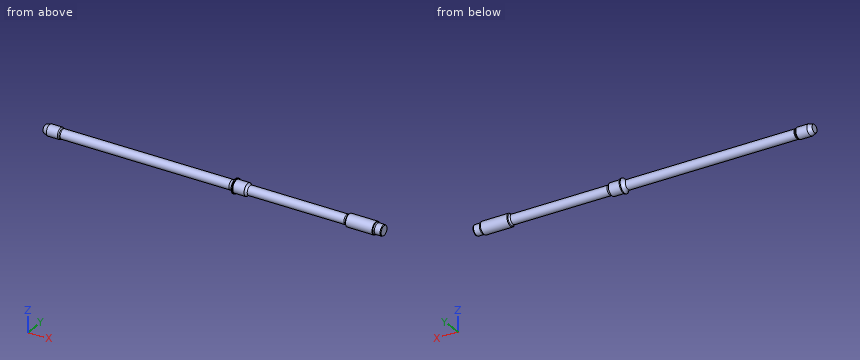
```python
from build123d import *

# Parameters (mm, degrees)
F4_R = 0.25
F5_R = 5
F6_R = 5


# Not quite as in the source:
# - a fillet or chamfer that OpenCascade refuses, or shapes differently, is made with other operations: its cross-section is extruded or revolved along the edge and cut away or added


with BuildPart() as f1:
    # F0 (on Front) → F1 (revolve)
    with BuildSketch(Plane.XZ):
        with BuildLine():
            Line((-2, 9.525), (-350.6009565311, 9.525))
            Line((-350.6009565311, 9.525), (-354, 11.11))
            Line((-354, 11.11), (-376.25, 11.11))
            Line((-376.25, 11.11), (-385, 8))
            Line((-385, 8), (-385, 0))
            Line((-385, 0), (297.49, 0))
            Line((297.49, 0), (297.49, 9.6239745962))
            Line((297.49, 9.6239745962), (295.99, 10.49))
            Line((295.99, 10.49), (284.1809884429, 10.49))
            ThreePointArc((284.1809884429, 10.49), (282.8216403227, 10.297737003), (281.7297929543, 11.13))
            Line((281.7297929543, 11.13), (280.97, 12.446))
            Line((280.97, 12.446), (227.5, 12.446))
            Line((227.5, 12.446), (224.579, 9.525))
            Line((224.579, 9.525), (23, 9.525))
            Line((23, 9.525), (23, 12.495))
            Line((23, 12.495), (0, 12.495))
            Line((0, 12.495), (0, 14.35))
            Line((0, 14.35), (-2, 14.35))
            Line((-2, 14.35), (-2, 9.525))
        make_face()
    revolve(axis=Axis((-43.755, 0, 0), (-1, 0, 0)))

    # F2: fillet of radius 8 on 1 edges, made by hand

    # F2_s1 → F2_t2 (revolve)
    with BuildSketch(Plane.XZ):
        with BuildLine():
            ThreePointArc((-2, 14.35), (-4.9498048155, 10.8391941398), (-9.3429813428, 9.525))
            Line((-9.3429813428, 9.525), (-2, 9.525))
            Line((-2, 9.525), (-2, 14.35))
        make_face()
    revolve(axis=Axis((-2, 0, 0), (-1, 0, 0)))

    # F3: fillet of radius 5 on 1 edges, made by hand

    # F3_s1 → F3_t2 (revolve)
    with BuildSketch(Plane.XZ):
        with BuildLine():
            ThreePointArc((27.5693653826, 9.525), (24.8444800639, 10.3327452367), (23, 12.495))
            Line((23, 12.495), (23, 9.525))
            Line((23, 9.525), (27.5693653826, 9.525))
        make_face()
    revolve(axis=Axis((23, 0, 0), (-1, 0, 0)))

    # F4
    f4_edges = [f1.edges().sort_by_distance(p)[0] for p in [
        (0, 0, -12.495),
    ]]
    fillet(f4_edges, radius=F4_R)

    # F5
    f5_edges = [f1.edges().sort_by_distance(p)[0] for p in [
        (-350.600957, 0, -9.525),
    ]]
    fillet(f5_edges, radius=F5_R)

    # F6
    f6_edges = [f1.edges().sort_by_distance(p)[0] for p in [
        (224.579, 0, -9.525),
    ]]
    fillet(f6_edges, radius=F6_R)


solid = f1.part
```
The model under review builds one solid part; all positions refer to its coordinate system, in mm. Round coordinates to 2 decimals unless told otherwise and drop trailing zeros. Loops run counter-clockwise (first coordinate to the right, second up) from the corner with the lowest first, then second, coordinate; pieces in that order, holes last. Notation, with made-up numbers: (-33, 58) - (-11, 58) arc R23 ccw to (-11, 97) - close; hole circle Ø1 at (16, 7). An arc over 180 degrees is marked (long way). Write each question's results on one line, items separated by ' | '. Start each with the question number.
Q1. Wall thickness on line 1 along Z through (x, y) = (-47, 5); line 2 along X through (y, z) = (9, 5.25); line 3 along Z through (x, y) = (113.5, 0.25): over which ranges is each line inside the solid? List them lowest first. Write a range as [from, to].
Q2. Insertion check: P1, Ø2, axis at x = -209, y = 11.5, coming from the -Z side; P2, Ø2, axis at x = -250, z = -5, coming from the +Y side; P3, Ø8, axis at x = -226.5, y = 10, coming from the -Z side; P4, Ø1.5, axis at y = 11.5, z = -7.5, coming from the -X side. Each pin has a flat end and moves straight along its axis. Give the tip position at first contact, or say it passes through.
Q3. Take a section at A-A on x = -103. Give the boundary of the cut face in (y, z) (3 decimals), plus the area to 3 significant figures.
Data:
1) line 1: z = [-8.11, 8.11] | line 2: x = [-378.19, -352.52], [-5.67, 24.72], [225.36, 282.49], [284.05, 296.11] | line 3: z = [-9.52, 9.52]
2) P1: passes through | P2: stops at y = 8.64 | P3: stops at z = -7.4 | P4: stops at x = -2.76
3) outline: circle Ø19.05 at (0, 0) | area: 285 mm²
